Can you work these out from the model? Positions are in its coordinate system, mm. Give positions to 0.01 mm unless a question says otherwise; leave off trailing zeros. Loops run counter-clockwise (first coordinate to the right, second up) from the corner with the lowest first, then second, coordinate; pieces in that order, holes last. Notation, with made-up numbers: M 18.25,79 L 72.25,79 A35 ccw 72.25,117 Z; hole C -37.5,69 d1. An arc over 180 degrees is marked long. Put each result on its own line as item: value. Start each with the question number.
1) For P1, Ø2, axis at y = 1.5, z = 12.5, coming from the -X side; P2, Ø1, axis at x = 10, y = 2.5, coming from the +Z side, each with a flat end and sliding along its axis, tell me the tip position at first contact or that it passes through.
2) Imagine slicing it at C-C (z = -11). Write out the boundary of the cut face in (x, y) (3 decimals), then the cut area to 3 significant figures.
3) Please list where these lines run through material, in increasing order: line 1 along Z through (x, y) = (-1.25, 0); line 2 along X through (y, z) = (0, -16.5); line 3 along X through (y, z) = (2.5, -8). Write a range as from..to.
4) Imagine slicing it at B-B (x = 10). Write out the boundary of the cut face in (y, z) (3 decimals), then the cut area to 3 significant figures.
5) Imagine slicing it at D-D (y = 2.75). Write out the boundary of the cut face in (x, z).
6) Imagine slicing it at A-A (y = 0). Write out the boundary of the cut face in (x, z), then the cut area to 3 significant figures.
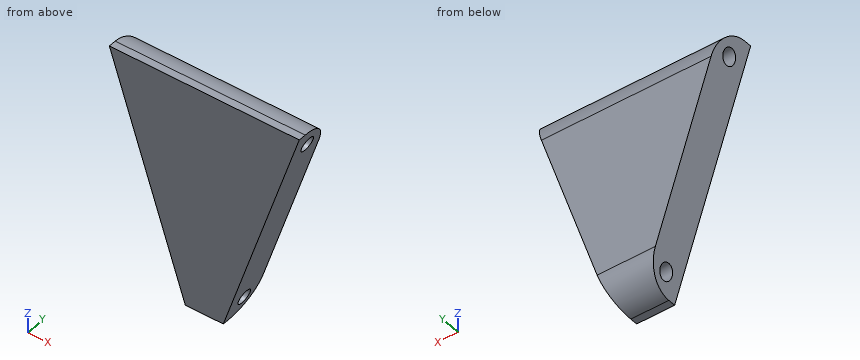
from build123d import *

# Parameters (mm, degrees)
F1_DEPTH = 3.175
F2_R     = 5.08
F3_R     = 1.27
F4_DEPTH = 25.4


with BuildPart() as f1:
    # F0 (on Front) → F1 (new body, symmetric)
    with BuildSketch(Plane.XZ):
        Polygon((15.851528, 17.014947), (-15.898472, 17.014947), (-3.198472, -21.085053), (3.151528, -21.085053), align=None)
    extrude(amount=F1_DEPTH, both=True)

    # F2
    f2_edges = [f1.edges().sort_by_distance(p)[0] for p in [
        (-0.023472, 3.175, 17.014947),
        (-0.023472, 3.175, -21.085053),
    ]]
    fillet(f2_edges, radius=F2_R)

    # F3 (on Right) → F4 (cut, symmetric)
    with BuildSketch(Plane.YZ):
        with Locations((0, 13.631148)):
            Circle(F3_R)
        with Locations((0, -17.971655)):
            Circle(F3_R)
    extrude(amount=F4_DEPTH, both=True, mode=Mode.SUBTRACT)


solid = f1.part
Recorded:
1. P1: x = -14.73
1. P2: z = 15.18
2. outline: M -6.56,-3.175 L 6.513,-3.175 L 6.513,3.175 L -6.56,3.175 Z
2. area: 83.0 mm²
3. line 1: -20.71..-19.24, -16.7..12.36, 14.9..16.64
3. line 2: -4.73..4.68
3. line 3: -7.56..7.51
4. outline: M -3.175,-0.54 L 3.175,-0.54 L 3.175,11.935 A5.08 ccw -1.905,17.015 L -3.175,17.015 Z; hole C 0,13.631 d2.54
4. area: 101 mm²
5. outline: M -14.88,13.97 L -4.21,-18.04 L 4.17,-18.04 L 14.84,13.97 Z
6. outline: M -15.77,16.64 L -15.19,14.9 L 15.15,14.9 L 15.73,16.64 Z; M -14.35,12.36 L -4.66,-16.7 L 4.61,-16.7 L 14.3,12.36 Z; M -3.81,-19.24 L -3.32,-20.71 L 3.28,-20.71 L 3.77,-19.24 Z
6. area: 615 mm²
